```python
from build123d import *

# Parameters (mm, degrees)
SKETCH1_W                         = 1409.7
SKETCH1_H                         = 76.2
BASE_FLANGE1_DEPTH                = 2.052574
EDGE_FLANGE1_DEPTH                = 1409.7
EDGE_FLANGE1_BEND_DEPTH           = 1409.7
SKETCH12_W                        = 76.2
SKETCH12_H                        = 25.4
CUT_EXTRUDE1_DEPTH                = 1414.376049374
F_9_START                         = -2.052574
F_9_0_196_DIAMETER_SLOT1_DEPTH    = 2.052574
F_10_0_1935_DIAMETER_HOLE1_D      = 4.9149
SKETCH18_W                        = 3.2639
SKETCH18_H                        = 84.252574
F_0_257_DIAMETER_HOLE1_AT_2_COUNT = 2
F_0_257_DIAMETER_HOLE1_AT_2_PITCH = 1308.1
F_0_257_DIAMETER_HOLE2_D          = 6.5278
FILLET1_R                         = 3.175


# Read off the part's stored shape, not the designer's step: #9 (0.196) Diameter Slot1
# Sheet-metal steps are written as plain solids
with BuildPart() as part:
    # Sketch1 → Base-Flange1 (new body)
    with BuildSketch(Plane(origin=(0, 0, 0), x_dir=(1, 0, 0), z_dir=(0, 1, 0))):
        with Locations((704.85, 38.1)):
            Rectangle(SKETCH1_W, SKETCH1_H)
    extrude(amount=-BASE_FLANGE1_DEPTH)

    # Edge-Flange1 section (across the edge) → Edge-Flange1 (add)
    with BuildSketch(Plane(origin=(0, 0, 3), x_dir=(0, 0, -1), z_dir=(1, 0, 0))):
        with BuildLine():
            Line((-2.052574, 3), (-2.052574, 61.447426))
            Line((-2.052574, 61.447426), (0, 61.447426))
            Line((0, 61.447426), (0, 3))
            ThreePointArc((0, 3), (0.878679656, 0.878679656), (3, 0))
            Line((3, 0), (3, -2.052574))
            ThreePointArc((3, -2.052574), (-0.572709338, -0.572709338), (-2.052574, 3))
        make_face()
    extrude(amount=EDGE_FLANGE1_DEPTH)

    # Edge-Flange1 section 2 (across the edge) → Edge-Flange1 bend (add)
    with BuildSketch(Plane(origin=(1409.7, 0, -79.2), x_dir=(0, 0, 1), z_dir=(-1, 0, 0))):
        with BuildLine():
            Line((-2.052574, 3), (-2.052574, 61.447426))
            Line((-2.052574, 61.447426), (0, 61.447426))
            Line((0, 61.447426), (0, 3))
            ThreePointArc((0, 3), (0.878679656, 0.878679656), (3, 0))
            Line((3, 0), (3, -2.052574))
            ThreePointArc((3, -2.052574), (-0.572709338, -0.572709338), (-2.052574, 3))
        make_face()
    extrude(amount=EDGE_FLANGE1_BEND_DEPTH)

    # Sketch12 → Cut-Extrude1 (cut, through all)
    with BuildSketch(Plane(origin=(0, 0, 0), x_dir=(1, 0, 0), z_dir=(0, 1, 0))):
        with Locations((1041.4, 38.1)):
            Rectangle(SKETCH12_W, SKETCH12_H)
    extrude(amount=-CUT_EXTRUDE1_DEPTH, mode=Mode.SUBTRACT)

    # #9 (0.196) Diameter Slot1 outline → #9 (0.196) Diameter Slot1 (cut)
    with BuildSketch(Plane(origin=(0, 0, 0), x_dir=(1, 0, 0), z_dir=(0, 1, 0)).offset(F_9_START)):
        with BuildLine():
            Line((1024.843257889, 59.59668), (1045.264857889, 59.59668))
            ThreePointArc((1045.264857889, 59.59668), (1047.754057889, 62.08588), (1045.264857889, 64.57508))
            Line((1045.264857889, 64.57508), (1024.843257889, 64.57508))
            ThreePointArc((1024.843257889, 64.57508), (1022.354057889, 62.08588), (1024.843257889, 59.59668))
        make_face()
        with BuildLine():
            ThreePointArc((1077.0108, 59.59668), (1079.5, 62.08588), (1077.0108, 64.57508))
            Line((1077.0108, 64.57508), (1056.5892, 64.57508))
            ThreePointArc((1056.5892, 64.57508), (1054.1, 62.08588), (1056.5892, 59.59668))
            Line((1056.5892, 59.59668), (1077.0108, 59.59668))
        make_face()
        with BuildLine():
            Line((1024.843257889, 11.117318322), (1045.264857889, 11.117318322))
            ThreePointArc((1045.264857889, 11.117318322), (1047.754057889, 13.606518322), (1045.264857889, 16.095718322))
            Line((1045.264857889, 16.095718322), (1024.843257889, 16.095718322))
            ThreePointArc((1024.843257889, 16.095718322), (1022.354057889, 13.606518322), (1024.843257889, 11.117318322))
        make_face()
        with BuildLine():
            Line((1056.5892, 11.62492), (1077.0108, 11.62492))
            ThreePointArc((1077.0108, 11.62492), (1079.5, 14.11412), (1077.0108, 16.60332))
            Line((1077.0108, 16.60332), (1056.5892, 16.60332))
            ThreePointArc((1056.5892, 16.60332), (1054.1, 14.11412), (1056.5892, 11.62492))
        make_face()
    extrude(amount=F_9_0_196_DIAMETER_SLOT1_DEPTH, mode=Mode.SUBTRACT)

    # #10 (0.1935) Diameter Hole1 (through all)
    with Locations(Plane(origin=(0, 0, -81.252574), x_dir=(-1, 0, 0), z_dir=(0, 0, -1))):
        with Locations((-1384.3, 29.697426), (-1333.5, 29.697426), (-1231.9, 29.697426), (-1181.1, 29.697426), (-228.6, 29.697426), (-177.8, 29.697426), (-76.2, 29.697426), (-25.4, 29.697426)):
            Hole(F_10_0_1935_DIAMETER_HOLE1_D / 2)

    # Sketch18 → F (0.257) Diameter Hole1 (revolve, cut)
    with BuildSketch(Plane(origin=(1358.9, 48.229266, -79.2), x_dir=(0, 1, 0), z_dir=(1, 0, 0))):
        with Locations((1.63195, 42.126287)):
            Rectangle(SKETCH18_W, SKETCH18_H)
    f_0_257_diameter_hole1 = revolve(axis=Axis((1358.9, 48.229266, -85.55), (0, 0, 1)), mode=Mode.SUBTRACT)

    # F (0.257) Diameter Hole1 at 2: F (0.257) Diameter Hole1 ×2
    with Locations(*[(-i * F_0_257_DIAMETER_HOLE1_AT_2_PITCH, 0, 0) for i in range(1, F_0_257_DIAMETER_HOLE1_AT_2_COUNT)]):
        add(f_0_257_diameter_hole1, mode=Mode.SUBTRACT)

    # F (0.257) Diameter Hole2 (through all)
    with Locations(Plane.XY.offset(-79.2)):
        with Locations((50.8, 48.229266), (1358.9, 48.229266)):
            Hole(F_0_257_DIAMETER_HOLE2_D / 2)

    # Fillet1
    fillet1_edges = [part.edges().sort_by_distance(p)[0] for p in [
        (0, 61.447426, 4.026287),
        (1409.7, 61.447426, 4.026287),
        (1409.7, 61.447426, -80.226287),
        (0, 61.447426, -80.226287),
    ]]
    fillet(fillet1_edges, radius=FILLET1_R)


solid = part.part
```
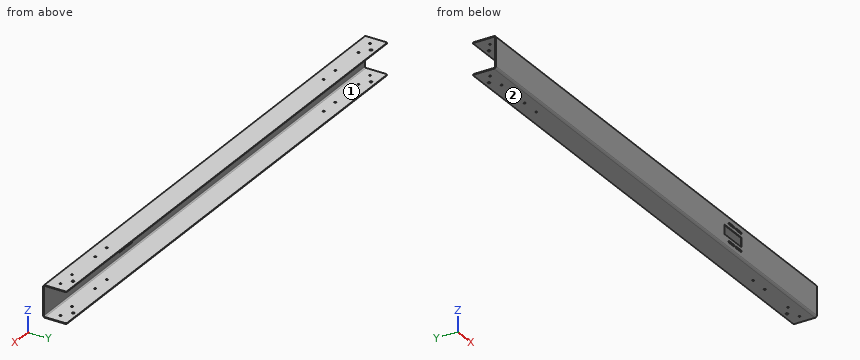
Can you work these out from the model? Positions are in its coordinate system, mm. Face numbers are marked on the shaded views. A direction names the side the tool comes from. Coordinates: 2 decimals unless noted, no trailing zeros. Loops run counter-clockwise (first coordinate to the right, second up) from the corner with the lowest first, then second, coordinate; pieces in that order, holes last. Notation, with made-up numbers: M 80,-2.5 L 95,-2.5 A16 ccw 95,10.5 Z; hole C 36,-21 d2. An arc over 180 degrees is marked long. Put each result on its own line as item: value. Start each with the question number.
(1) Imagine slicing it at A-A on x = 795. List the corners of the cut face in (y, z) for me, and give its area (3 significant figures).
(2) I need wall thicknesses on probe 1 along Z at (x, y) = (514, 18.5); probe 2 along Y at (x, z) = (821, -50); probe 3 along Y at (x, z) = (50.8, -80.5). Which ranges of each line are inside material? Lowest first, please.
(3) Will these pins go through, and if not, where does the flat tip stop? pin 1 Ø1 at (x, y) = (1064, -1) entering from -Z; pin 2 Ø2.5 at (y, z) = (-0.5, -44) entering from -X; pin 3 Ø0.6 at (x, y) = (1029.5, -1) entering from +Z; pin 4 Ø2 at (x, z) = (483.5, -26.5) entering from +Y.
(4) Which directions (+Z, -Z, +X, -X, +Y, -Y) give clear straight access to the entire face, cutting with the end or side of a thin tool? Please do the marked faces 1 and 2.
Worked answers:
1. outline: M -2.05,-76.2 A5.05 ccw 3,-81.25 L 61.45,-81.25 L 61.45,-79.2 L 3,-79.2 A3 cw 0,-76.2 L 0,0 A3 cw 3,3 L 61.45,3 L 61.45,5.05 L 3,5.05 A5.05 ccw -2.05,0 Z
1. area: 422 mm2
2. probe 1: z = -81.25 to -79.2, 3 to 5.05
2. probe 2: y = -2.05 to 0
2. probe 3: y = 0.35 to 44.97, 51.49 to 61.45
3. pin 1: stops at z = -79.84
3. pin 2: stops at x = 0
3. pin 3: stops at z = 3.44
3. pin 4: stops at y = 0
4. face 1: +X, -X, +Y
4. face 2: -Z, +X, -X, +Y, -Y
